Geometry: final body of the model. Coordinates: model frame, mm. A direction names the side the tool comes from. Give positions to 0.01 mm unless a question says otherwise; leave off trailing zeros. Order: outer loops, then holes, each group sorted by start corner. A loop starts at its lowest first (then second) coordinate and runs counter-clockwise, first axis right, second up. Notation, with made-up numbers: (35, 86.5) - (67, 86.5) arc R7 ccw to (67, 94.5) - close; hole circle Ø10 at (-11, 43). An arc over 180 degrees is marked (long way). Put each result on its own line as item: value. Start each with the question number.
1. Mould query, pull axis X, two halves, no side actions, for faces 4 (the flat face through (7, 1, 0.973)), 5 (the flat face through (60.541, 1, -2)), 6 (the flat face through (-10, 1, -8.752)). Classes: pulls with the +X half, pulls with the -X half, needs draft (parallel to the pull), parting line crosses it, or undercut.
2. Section C-C on z = 6.75. Return the cut outline in (x, y), plus the area to 3 significant figures.
3. Section B-B on x = 38. Return the cut outline in (y, z), plus the area to 3 significant figures.
4. Set-up query: faces 1 (the flat face through (34, 1, 5.091)), 2 (the flat face through (38, 1, -5.069)), 3 (the flat face through (14.115, 1, -2)). Return all of +Z, -Z, +X, -X, +Y, -Y with unobstructed straight access to the full face (end or side cutting, diameter ignored); none if empty.
5. First-contact query: P1, Ø0.8, axis at x = 38.5, y = 1.5, coming from the +Z side. Flat tip, straight axial feed; report the tip coordinate or a pass-through.
6. Section A-A on y = 1.4. Return the cut outline in (x, z), plus the area to 3 significant figures.
7. Ray query, line 1 along X through (y, z) = (1.55, -0.75); line 2 along X through (y, z) = (1.3, -5.5); line 3 along X through (y, z) = (0.7, -2). Return the intervals inside material, ascending. Write a range as from..to.
from build123d import *

# Parameters (mm, degrees)
SKETCH1_R           = 1.016
SKETCH1_R_2         = 1.600000102
SKETCH1_R_3         = 1.0922
BOSS_EXTRUDE1_DEPTH = 2.54
SKETCH2_W           = 13.66210268
SKETCH2_H           = 9.772536081
CUT_EXTRUDE1_DEPTH  = 2.54


with BuildPart() as part:
    # Sketch1 → Boss-Extrude1 (new body)
    with BuildSketch(Plane(origin=(0, 0, 0), x_dir=(1, 0, 0), z_dir=(0, 1, 0))):
        Polygon((-13.753823011, 8.752244808), (-13.753823011, 2.783244808), (-13.753823011, -5.090755192), (-10.551287224, -9.623078218), (8.47904741, -9.623078218), (21.176501094, -5.090755192), (33.876501094, -5.090755192), (47.455454133, -5.090755192), (60.541176989, -0.789612996), (60.541176989, -0.010755192), (60.541176989, 5.069244808), (37.046176989, 5.069244808), (25.616176989, 5.069244808), (13.567051989, 5.069244808), (-7.149823011, 8.752244808), align=None)
        with Locations(Location((22.441176989, 2.529244808, 0), (0, 0, 270))):
            Circle(SKETCH1_R, mode=Mode.SUBTRACT)
        with Locations(Location((55.461176989, 2.529244808, 0), (0, 0, 270))):
            Circle(SKETCH1_R_2, mode=Mode.SUBTRACT)
        with Locations(Location((-10.578823011, 5.323244808, 0), (0, 0, 270))):
            Circle(SKETCH1_R_2, mode=Mode.SUBTRACT)
        with Locations(Location((43.278107208, 2.529244808, 0), (0, 0, 270))):
            Circle(SKETCH1_R_3, mode=Mode.SUBTRACT)
    extrude(amount=BOSS_EXTRUDE1_DEPTH)

    # Sketch2 → Cut-Extrude1 (cut)
    with BuildSketch(Plane.XZ):
        with Locations((7.284233537, -3.91320906)):
            Rectangle(SKETCH2_W, SKETCH2_H)
    extrude(amount=-CUT_EXTRUDE1_DEPTH, mode=Mode.SUBTRACT)


solid = part.part
Resolved:
1. face 4: undercut
1. face 5: pulls with the +X half
1. face 6: needs draft
2. outline: (-12.58, 0) - (16.53, 0) - (16.53, 2.54) - (-12.58, 2.54) - close
2. area: 73.9 mm^2
3. outline: (0, -5.07) - (2.54, -5.07) - (2.54, 5.09) - (0, 5.09) - close
3. area: 25.8 mm^2
4. face 1: +Z, +X, +Y, -Y
4. face 2: -Z, +X, +Y, -Y
4. face 3: -Z, +Y, -Y
5. P1: z = 5.09
6. outline: (-13.75, -8.75) - (-7.15, -8.75) - (0.45, -7.4) - (0.45, 0.97) - (14.12, 0.97) - (14.12, -5.07) - (60.54, -5.07) - (60.54, 0.79) - (47.46, 5.09) - (21.18, 5.09) - (8.48, 9.62) - (-10.55, 9.62) - (-13.75, 5.09) - close; hole circle Ø3.2 at (-10.58, -5.32); hole circle Ø2.03 at (22.44, -2.53); hole circle Ø2.18 at (43.28, -2.53); hole circle Ø3.2 at (55.46, -2.53)
6. area: 791 mm^2
7. line 1: -13.75..0.45, 14.12..60.54
7. line 2: -13.75..-12.17, -8.99..0.45
7. line 3: -13.75..0.45, 14.12..21.57, 23.31..42.32, 44.23..53.95, 56.97..60.54
